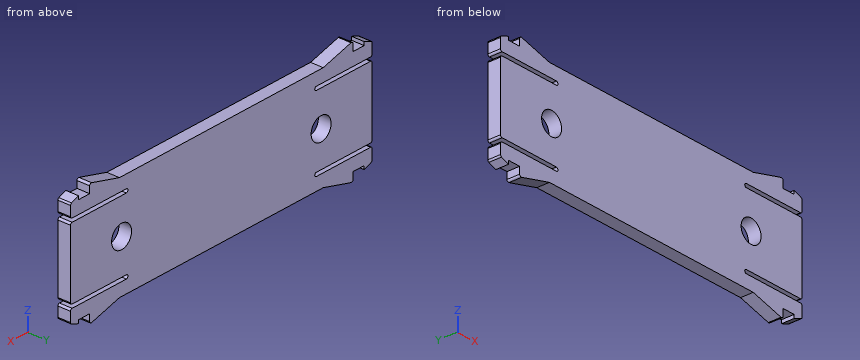
from build123d import *

# Parameters (mm, degrees)
PAD010_DEPTH    = 2.8
FILLET003_R     = 0.4
SKETCH016_R     = 2.5
POCKET008_DEPTH = 2.801


with BuildPart() as part:
    # Sketch010 (on Face2 of ShapeBinder009) → Pad010 (new body)
    with BuildSketch(Plane.XZ.offset(25.388718)):
        with BuildLine():
            Line((37.8, 63.127675), (37.8, 60.327675))
            Line((37.8, 60.327675), (23.8, 60.327675))
            ThreePointArc((23.8, 60.327675), (23.4, 59.927675), (23.8, 59.527675))
            Line((23.8, 59.527675), (37.8, 59.527675))
            Line((37.8, 59.527675), (37.8, 44.127675))
            Line((37.8, 44.127675), (23.8, 44.127675))
            ThreePointArc((23.8, 44.127675), (23.4, 43.727675), (23.8, 43.327675))
            Line((23.8, 43.327675), (37.8, 43.327675))
            Line((37.8, 43.327675), (37.8, 40.527675))
            Line((37.8, 40.527675), (35.8, 39.777675))
            Line((35.8, 40.527675), (35.8, 39.777675))
            Line((35.8, 40.527675), (33, 40.527675))
            Line((33, 40.527675), (33, 38.527675))
            Line((33, 38.527675), (25.535898, 40.527675))
            Line((25.535898, 40.527675), (-25.535898, 40.527675))
            Line((-25.535898, 40.527675), (-33, 38.527675))
            Line((-33, 38.527675), (-33, 40.527675))
            Line((-33, 40.527675), (-35.8, 40.527675))
            Line((-35.8, 40.527675), (-35.8, 39.777675))
            Line((-37.8, 40.527675), (-35.8, 39.777675))
            Line((-37.8, 40.527675), (-37.8, 43.327675))
            Line((-37.8, 43.327675), (-23.8, 43.327675))
            ThreePointArc((-23.8, 43.327675), (-23.4, 43.727675), (-23.8, 44.127675))
            Line((-23.8, 44.127675), (-37.8, 44.127675))
            Line((-37.8, 44.127675), (-37.8, 59.527675))
            Line((-37.8, 59.527675), (-23.8, 59.527675))
            ThreePointArc((-23.8, 59.527675), (-23.4, 59.927675), (-23.8, 60.327675))
            Line((-23.8, 60.327675), (-37.8, 60.327675))
            Line((-37.8, 60.327675), (-37.8, 63.127675))
            Line((-35.8, 63.877675), (-37.8, 63.127675))
            Line((-35.8, 63.127675), (-35.8, 63.877675))
            Line((-35.8, 63.127675), (-33, 63.127675))
            Line((-33, 63.127675), (-33, 65.127675))
            Line((-33, 65.127675), (-25.535898, 63.127675))
            Line((-25.535898, 63.127675), (25.535898, 63.127675))
            Line((25.535898, 63.127675), (33, 65.127675))
            Line((33, 65.127675), (33, 63.127675))
            Line((33, 63.127675), (35.8, 63.127675))
            Line((35.8, 63.127675), (35.8, 63.877675))
            Line((35.8, 63.877675), (37.8, 63.127675))
        make_face()
    extrude(amount=-PAD010_DEPTH)

    # Fillet003
    fillet003_edges = [part.edges().sort_by_distance(p)[0] for p in [
        (33, -23.988718, 65.127675),
        (37.8, -23.988718, 63.127675),
        (37.8, -23.988718, 60.327675),
        (37.8, -23.988718, 59.527675),
        (37.8, -23.988718, 44.127675),
        (37.8, -23.988718, 43.327675),
        (37.8, -23.988718, 40.527675),
        (33, -23.988718, 38.527675),
        (-33, -23.988718, 65.127675),
        (-37.8, -23.988718, 63.127675),
        (-37.8, -23.988718, 60.327675),
        (-37.8, -23.988718, 59.527675),
        (-37.8, -23.988718, 44.127675),
        (-37.8, -23.988718, 43.327675),
        (-37.8, -23.988718, 40.527675),
        (-33, -23.988718, 38.527675),
    ]]
    fillet(fillet003_edges, radius=FILLET003_R)

    # Sketch016 (on Face2 of Fillet003) → Pocket008 (cut, through all)
    with BuildSketch(Plane.XZ.offset(25.388718)):
        with Locations((-25, 51.827675)):
            Circle(SKETCH016_R)
        with Locations((25, 51.827675)):
            Circle(SKETCH016_R)
    extrude(amount=-POCKET008_DEPTH, mode=Mode.SUBTRACT)


solid = part.part
For this review, take the finished solid that the model builds, in its own axes (mm). Round coordinates to 2 decimals unless told otherwise and drop trailing zeros. Write each loop counter-clockwise with the first axis right and the second up, starting at its lowest first coordinate (ties: lowest second). Pieces come first, ordered by that corner, then holes. Notation, with made-up numbers: (85.25, 43) -> (137.25, 43) arc R30 cw to (137.25, 82) -> close; hole circle Ø10 at (-30, 63). An arc over 180 degrees is marked (long way). Put each result on its own line as item: value.
Q1. Consider section A-A on z = 50.75. State the section outline as (x, y) points, and give its area (3 significant figures).
Determined:
outline: (-37.8, -25.39) -> (-27.26, -25.39) -> (-27.26, -22.59) -> (-37.8, -22.59) -> close; (-22.74, -25.39) -> (22.74, -25.39) -> (22.74, -22.59) -> (-22.74, -22.59) -> close; (27.26, -25.39) -> (37.8, -25.39) -> (37.8, -22.59) -> (27.26, -22.59) -> close
area: 186 mm^2
Q2. Consider section C-C on x = 26.5. State the section outline as (y, z) points.
Determined:
outline: (-25.39, 40.27) -> (-22.59, 40.27) -> (-22.59, 43.33) -> (-25.39, 43.33) -> close; (-25.39, 44.13) -> (-22.59, 44.13) -> (-22.59, 49.83) -> (-25.39, 49.83) -> close; (-25.39, 53.83) -> (-22.59, 53.83) -> (-22.59, 59.53) -> (-25.39, 59.53) -> close; (-25.39, 60.33) -> (-22.59, 60.33) -> (-22.59, 63.39) -> (-25.39, 63.39) -> close
Q3. Consider section B-B on x = -30. State the section outline as (y, z) points, and give its area (3 significant figures).
Determined:
outline: (-25.39, 39.33) -> (-22.59, 39.33) -> (-22.59, 43.33) -> (-25.39, 43.33) -> close; (-25.39, 44.13) -> (-22.59, 44.13) -> (-22.59, 59.53) -> (-25.39, 59.53) -> close; (-25.39, 60.33) -> (-22.59, 60.33) -> (-22.59, 64.32) -> (-25.39, 64.32) -> close
area: 65.5 mm^2
Q4. Consider section D-D on x = -18. State the section outline as (y, z) points, and give its area (3 significant figures).
Determined:
outline: (-25.39, 40.53) -> (-22.59, 40.53) -> (-22.59, 63.13) -> (-25.39, 63.13) -> close
area: 63.3 mm^2
Q5. To check wall thickness, follow L1, parallel to Z at x = 25, y = -24; L2, parallel to X at y = -23.7, z = 51.5; L3, parallel to X at y = -25, z = 50. State the ranges of each line that lie inside material, in increasing order. Write a range as [from, to].
Determined:
L1: z = [40.53, 43.33], [44.13, 49.33], [54.33, 59.53], [60.33, 63.13]
L2: x = [-37.8, -27.48], [-22.52, 22.52], [27.48, 37.8]
L3: x = [-37.8, -26.71], [-23.29, 23.29], [26.71, 37.8]
Q6. Clearance check with flat-ended pins moving along their axes: pin 1 Ø0.8 at (x, y) = (34.5, -24.5) entering from -Z; pin 2 Ø1.4 at (x, y) = (35, -24) entering from +Z; pin 3 Ø1.4 at (x, y) = (-27.5, -23.5) entering from -Z; pin 4 Ø6.5 at (x, z) = (25, 51.83) entering from -Y. State where each tip first meets the part, or that it passes through.
Determined:
pin 1: stops at z = 40.53
pin 2: stops at z = 63.13
pin 3: stops at z = 39.81
pin 4: stops at y = -25.39
